```python
from build123d import *

# Parameters (mm, degrees)
SKETCH3_R          = 1.1
CUT_EXTRUDE1_DEPTH = 6
CIRPATTERN1_COUNT  = 8
CHAMFER2_SIZE      = 1.25
CHAMFER2_SIZE2     = 2.165063509


with BuildPart() as part:
    # Sketch2 → Revolve1 (revolve)
    with BuildSketch(Plane.XY, mode=Mode.PRIVATE) as revolve1_sk:
        Polygon((-2.5, 0), (-2.5, 2), (-8, 17), (-10.9, 17), (-10.9, 2), (-10.9, -1), (-8.65, -1), (-8.65, -4.5), (-10.9, -4.5), (-10.9, -8.4), align=None)
    revolve(revolve1_sk.sketch.rotate(Axis((0, 19.141519074, 0), (0, -1, 0)), 270), axis=Axis((0, 19.141519074, 0), (0, -1, 0)))

    # Sketch3 → Cut-Extrude1 (cut)
    with BuildSketch(Plane.ZY.offset(10.9)):
        with Locations((0, 2)):
            Circle(SKETCH3_R)
    cut_extrude1 = extrude(amount=-CUT_EXTRUDE1_DEPTH, mode=Mode.SUBTRACT)

    # CirPattern1: Cut-Extrude1 ×8 about axis
    cirpattern1_axis = Axis((0, 0, 0), (0, 1, 0))
    for i in range(1, CIRPATTERN1_COUNT):
        add(cut_extrude1.rotate(cirpattern1_axis, i * 360 / CIRPATTERN1_COUNT), mode=Mode.SUBTRACT)

    # Chamfer2
    chamfer2_edges = [part.edges().sort_by_distance(p)[0] for p in [
        (0, -4.5, -10.9),
    ]]
    chamfer2_side = [part.faces().sort_by_distance(p)[0] for p in [
        (0, -6.45, -10.9),
    ]]
    chamfer(chamfer2_edges, length=CHAMFER2_SIZE, length2=CHAMFER2_SIZE2, reference=chamfer2_side[0])


solid = part.part
```
Here's how the part is built. I have some questions about the finished solid (model axes, mm). A direction names the side the tool comes from. Coordinates: 2 decimals unless noted, no trailing zeros. Loops run counter-clockwise (first coordinate to the right, second up) from the corner with the lowest first, then second, coordinate; pieces in that order, holes last. Notation, with made-up numbers: M -16,-24.75 L 43,-24.75 A21 cw 43,6.25 Z; hole C 21.5,-28.75 d5. An arc over 180 degrees is marked long. One line per item, written item: value.
1. Will these pins go through, and if not, where does the flat tip stop? pin 1 Ø4 at (x, y) = (-6.5, -4) entering from +Z; pin 2 Ø1.8 at (y, z) = (2, 0) entering from -X; pin 3 Ø4 at (y, z) = (0, -4.5) entering from +X.
Geometry says:
pin 1: stops at z = 9.39
pin 2: stops at x = -4.9
pin 3: stops at x = 10.61
2. Imagine slicing it at C-C (y = -2.75). List the corners of the cut face in (x, z) for me.
Geometry says:
outline: C 0,0 d17.3; hole C 0,0 d10.5
3. Imagine slicing it at A-A (x = 0). List the corners of the cut face in (y, z) for me, and give its area (3 significant figures).
Geometry says:
outline: M -8.4,-10.9 L -5.75,-10.9 L -4.5,-8.73 L -4.5,-8.65 L -1,-8.65 L -1,-10.9 L 0.9,-10.9 L 0.9,-4.9 L 3.1,-4.9 L 3.1,-10.9 L 17,-10.9 L 17,-8 L 2,-2.5 L 0,-2.5 Z; M -8.4,10.9 L 0,2.5 L 2,2.5 L 17,8 L 17,10.9 L 3.1,10.9 L 3.1,4.9 L 0.9,4.9 L 0.9,10.9 L -1,10.9 L -1,8.65 L -4.5,8.65 L -4.5,8.73 L -5.75,10.9 Z
area: 229 mm2
4. Thinking about a two-plate mould opening in Z: for faces 1 (the flat face through (0, 2, 4.9)), 2 (the cylindrical face through (10.64, -7.09, -2.36)), 3 (the flat face through (-6, 17, 6)), 4 (the cylindrical face through (4.897, 1.579, -6.334)), which applies, +Z half, -Z half, draft (parallel to the pull), parting line (faces both ways), or undercut?
Geometry says:
face 1: +Z half
face 2: parting line
face 3: draft
face 4: undercut
5. Please list where these lines run through material, in increasing order: probe 1 along X at (y, z) = (2, 6.75); probe 2 along X at (y, z) = (1.45, 0); probe 3 along Z at (x, y) = (9, 2).
Geometry says:
probe 1: x = -8.56 to -8.31, -5.19 to -1.1, 1.1 to 5.19, 8.31 to 8.56
probe 2: x = -4.9 to -2.5, 2.5 to 4.9
probe 3: z = -6.15 to -1.1, 1.1 to 6.15
6. Imagine slicing it at D-D (y = 7). List the corners of the cut face in (x, z) for me.
Geometry says:
outline: C 0,0 d21.8; hole C 0,0 d8.67
7. On a 3-axis mill with a long thin cutter (end or side, diameter ignored), from which of +Z, -Z, +X, -X, +Y, -Y can I reach the whole of each face in a straight line? I mean faces 5 (the flat face through (4.9, 2, 0)), 6 (the flat face through (-4.9, 2, 0)), 7 (the flat face through (3.48, 2.02, -3.45)), 8 (the cylindrical face through (0.238, 0.926, -7.942)), 9 (the cylindrical face through (-0.238, 0.926, 7.942)). Say none if no direction works.
Geometry says:
face 5: +X
face 6: -X
face 7: none
face 8: -Z
face 9: +Z
8. Imagine slicing it at B-B (z = 0). List the corners of the cut face in (x, y) for me.
Geometry says:
outline: M -10.9,-8.4 L -2.5,0 L -2.5,2 L -8,17 L -10.9,17 L -10.9,3.1 L -4.9,3.1 L -4.9,0.9 L -10.9,0.9 L -10.9,-1 L -8.65,-1 L -8.65,-4.5 L -8.73,-4.5 L -10.9,-5.75 Z; M 2.5,0 L 10.9,-8.4 L 10.9,-5.75 L 8.73,-4.5 L 8.65,-4.5 L 8.65,-1 L 10.9,-1 L 10.9,0.9 L 4.9,0.9 L 4.9,3.1 L 10.9,3.1 L 10.9,17 L 8,17 L 2.5,2 Z
